The listing builds one solid part. Answer for the finished solid, in the listing's coordinates (mm). A direction names the side the tool comes from. Round coordinates to 2 decimals unless told otherwise and drop trailing zeros. Order: outer loops, then holes, each group sorted by start corner. A loop starts at its lowest first (then second) coordinate and runs counter-clockwise, first axis right, second up. Notation, with made-up numbers: (57, 75) - (109, 75) arc R13 ccw to (109, 90) - close; hole circle Ø11 at (34.25, 88). An arc over 180 degrees is marked (long way). One line per item, written item: value. Start each with the question number.
1. Flat-ended cylindrical pins translate along their axes: P1, Ø3, axis at x = -29.545, y = 6.94, coming from the -Z side; P2, Ø2, axis at x = -38.5, y = 5, coming from the +Z side; P3, Ø4, axis at y = 9, z = 13.5, coming from the -X side; P4, Ø1, axis at y = 8.5, z = 5.5, coming from the +X side. Find the tip coordinate at first contact, or state that the pin passes through.
2. Section A-A, the plane x = -6 is taken. Give the vertices of the cut face in (y, z), then the cut area to 3 significant figures.
3. Section B-B, the plane y = 6 is taken. Count the separate pieces of the cut face and the enclosed holes in it, then the cut area to 3 significant figures.
4. A tool of negligible diameter and unlimited length cuts with its end or side. For faces 1 (the flat face through (-8, 4, 11.59)), 2 (the flat face through (-19, 0, 6)), from which of +Z, -Z, +X, -X, +Y, -Y can it reach the whole face along a straight path? Write none if from no direction.
5. Section D-D, the plane x = -27 is taken. Give the vertices of the cut face in (y, z), then the cut area to 3 significant figures.
6. Straight lines are drawn through the part: line 1 (Z direction, x = -12, y = 4.75); line 2 (Z direction, x = -43.5, y = 3.5); line 3 (Z direction, x = -17, y = 3). For each, find the intervals that lie inside material, in ascending order.
7. For a pull along X with two mould halves and no side action, classify faces 3 (the cylindrical face through (-18.813, 5.075, 7.94)), 4 (the flat face through (-4.9, 3.8, 4.52)), 5 (the flat face through (-49.85, 5, 2)) as released by +X, released by -X, zero draft, split by the parting line, or undercut.
8. Section C-C, the plane y = 2.75 is taken. Give the vertices of the cut face in (x, z) (3 decimals).
from build123d import *

# Parameters (mm, degrees)
BOSS_EXTRUDE1_DEPTH = 10.01
SKETCH2_R           = 4
CUT_EXTRUDE1_DEPTH  = 11.01
SKETCH3_R           = 1.6
CUT_EXTRUDE2_DEPTH  = 17.11
CUT_EXTRUDE3_REACH  = 18.11
SKETCH5_R           = 1.4


with BuildPart() as part:
    # Sketch1 → Boss-Extrude1 (new body)
    with BuildSketch(Plane(origin=(0, 0, 0), x_dir=(1, 0, 0), z_dir=(0, 1, 0))):
        with BuildLine():
            Line((-49.85, 0), (0, 0))
            Line((0, 0), (0, -4.52))
            Line((0, -4.52), (-14.815, -4.52))
            ThreePointArc((-14.815, -4.52), (-18.35, -8.055), (-14.815, -11.59))
            Line((-14.815, -11.59), (0, -11.59))
            Line((0, -11.59), (0, -16.11))
            Line((0, -16.11), (-14.815, -16.11))
            ThreePointArc((-14.815, -16.11), (-21.647183033, -12.32164974), (-22.052872616, -4.52))
            Line((-22.052872616, -4.52), (-49.85, -4.52))
            Line((-49.85, -4.52), (-49.85, 0))
        make_face()
    extrude(amount=BOSS_EXTRUDE1_DEPTH)

    # Sketch2 → Cut-Extrude1 (cut, through all)
    with BuildSketch(Plane(origin=(0, 10.01, 0), x_dir=(1, 0, 0), z_dir=(0, 1, 0))):
        with Locations((-14.815, -8.055)):
            Circle(SKETCH2_R)
    extrude(amount=-CUT_EXTRUDE1_DEPTH, mode=Mode.SUBTRACT)

    # Sketch3 → Cut-Extrude2 (cut, through all)
    with BuildSketch(Plane(origin=(0, 0, 0), x_dir=(-1, 0, 0), z_dir=(0, 0, -1))):
        with Locations((6.39994888, 5.005)):
            Circle(SKETCH3_R)
    extrude(amount=-CUT_EXTRUDE2_DEPTH, mode=Mode.SUBTRACT)

    # Sketch5 → Cut-Extrude3 (cut, up to next)
    with BuildSketch(Plane(origin=(0, 0, 0), x_dir=(-1, 0, 0), z_dir=(0, 0, -1)), mode=Mode.PRIVATE) as cut_extrude3_sk1:
        with Locations((29.545, 6.94)):
            Circle(SKETCH5_R)
    cut_extrude3_tool1 = extrude(cut_extrude3_sk1.sketch, amount=-CUT_EXTRUDE3_REACH, mode=Mode.PRIVATE) & part.part
    add(cut_extrude3_tool1.solids().sort_by_distance((-29.545, 6.94, 0))[0], mode=Mode.SUBTRACT)
    # Sketch5 → Cut-Extrude3 (cut, up to next)
    with BuildSketch(Plane(origin=(0, 0, 0), x_dir=(-1, 0, 0), z_dir=(0, 0, -1)), mode=Mode.PRIVATE) as cut_extrude3_sk2:
        with Locations((38.865, 6.94)):
            Circle(SKETCH5_R)
    cut_extrude3_tool2 = extrude(cut_extrude3_sk2.sketch, amount=-CUT_EXTRUDE3_REACH, mode=Mode.PRIVATE) & part.part
    add(cut_extrude3_tool2.solids().sort_by_distance((-38.865, 6.94, 0))[0], mode=Mode.SUBTRACT)


solid = part.part
Answer list:
1. P1: stops at z = 0
1. P2: stops at z = 4.52
1. P3: stops at x = -22.1
1. P4: stops at x = -17.4
2. outline: (0, 0) - (3.46, 0) - (3.46, 4.52) - (0, 4.52) - close; (0, 11.59) - (3.46, 11.59) - (3.46, 16.11) - (0, 16.11) - close; (6.55, 0) - (10.01, 0) - (10.01, 4.52) - (6.55, 4.52) - close; (6.55, 11.59) - (10.01, 11.59) - (10.01, 16.11) - (6.55, 16.11) - close
2. area: 62.5 mm²
3. separate pieces: 5
3. enclosed holes: 0
3. area: 303 mm²
4. face 1: +X, +Y, -Y
4. face 2: +Z, -Z, +X, -X, -Y
5. outline: (0, 0) - (10.01, 0) - (10.01, 4.52) - (0, 4.52) - close
5. area: 45.2 mm²
6. line 1: z = 0 to 4.52, 11.59 to 16.11
6. line 2: z = 0 to 4.52
6. line 3: z = 0 to 4.7, 11.41 to 15.81
7. face 3: undercut
7. face 4: zero draft
7. face 5: released by -X
8. outline: (-49.85, 0) - (0, 0) - (0, 4.52) - (-12.943, 4.52) arc R4 cw (long way) to (-12.943, 11.59) - (0, 11.59) - (0, 16.11) - (-14.815, 16.11) arc R8.055 ccw to (-22.053, 4.52) - (-49.85, 4.52) - close
